Here's how the part is built. I have some questions about the finished solid (model axes, mm). Face numbers are marked on the shaded views. A direction names the side the tool comes from. Give positions to 0.01 mm unless a question says otherwise; leave off trailing zeros. Write each loop counter-clockwise with the first axis right and the second up, starting at its lowest first coordinate (ties: lowest second). Pieces come first, ordered by that corner, then holes. Notation, with made-up numbers: (64, 50.5) - (85, 50.5) arc R31 cw to (85, 78.5) - close; hole circle Ø4 at (51, 84). An arc over 180 degrees is marked (long way). Use a Markdown table: item, result.
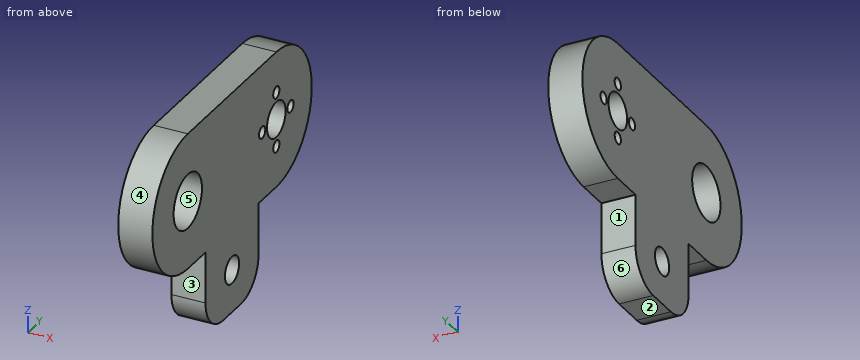
```python
from build123d import *

# Parameters (mm, degrees)
CROQUIS1_R              = 5.25
CROQUIS1_R_2            = 8
CROQUIS1_R_3            = 1.75
CROQUIS1_R_4            = 4
SALIENTE_EXTRUIR1_DEPTH = 10


with BuildPart() as part:
    # Croquis1 → Saliente-Extruir1 (new body)
    with BuildSketch(Plane(origin=(0, 0, 0), x_dir=(0, 0, -1), z_dir=(1, 0, 0))):
        with BuildLine():
            Line((20, 15), (20, 25))
            ThreePointArc((20, 25), (0, 45), (-20, 25))
            Line((-20, 25), (-20, -25))
            ThreePointArc((-20, -25), (0, -45), (20, -25))
            Line((20, -25), (20, -15))
            Line((20, -15), (35, -15))
            ThreePointArc((35, -15), (42.071067812, -12.071067812), (45, -5))
            Line((45, -5), (45, 5))
            ThreePointArc((45, 5), (42.071067812, 12.071067812), (35, 15))
            Line((35, 15), (20, 15))
        make_face()
        with Locations((0, 25)):
            Circle(CROQUIS1_R, mode=Mode.SUBTRACT)
        with Locations((0, -25)):
            Circle(CROQUIS1_R_2, mode=Mode.SUBTRACT)
        with Locations((0, 33)):
            Circle(CROQUIS1_R_3, mode=Mode.SUBTRACT)
        with Locations((8, 25)):
            Circle(CROQUIS1_R_3, mode=Mode.SUBTRACT)
        with Locations((0, 17)):
            Circle(CROQUIS1_R_3, mode=Mode.SUBTRACT)
        with Locations((-8, 25)):
            Circle(CROQUIS1_R_3, mode=Mode.SUBTRACT)
        with Locations((32.5, 0)):
            Circle(CROQUIS1_R_4, mode=Mode.SUBTRACT)
    extrude(amount=SALIENTE_EXTRUIR1_DEPTH)


solid = part.part
```
Item 1: If we section it at A-A, the plane y = 0: Write out the boundary of the cut face in (x, z).
Values:
| item | result |
|---|---|
| outline | (0, -45) - (10, -45) - (10, -36.5) - (0, -36.5) - close; (0, -28.5) - (10, -28.5) - (10, 20) - (0, 20) - close |
Item 2: I need wall thicknesses on line 1 along Y through (x, z) = (8, 0); line 2 along Z through (x, y) = (6.75, 16.5); line 3 along Z through (x, y) = (9, 29). Which ranges of each line are inside material? Lowest first, please. Write a range as [from, to].
Values:
| item | result |
|---|---|
| line 1 | y = [-45, -33], [-17, 15.25], [18.75, 19.75], [30.25, 31.25], [34.75, 45] |
| line 2 | z = [-20, -1.68], [1.68, 20] |
| line 3 | z = [-19.6, -3.4], [3.4, 19.6] |
Item 3: Will these pins go through, and if not, where does the flat tip stop? pin 1 Ø13 at (y, z) = (0, -32.5) entering from -X; pin 2 Ø2 at (x, y) = (8.5, -32) entering from +Z; pin 3 Ø4 at (x, z) = (2, 13) entering from -Y; pin 4 Ø5 at (x, y) = (3.5, 21) entering from -Z.
Values:
| item | result |
|---|---|
| pin 1 | stops at x = 0 |
| pin 2 | stops at z = 19.08 |
| pin 3 | stops at y = -41.7 |
| pin 4 | stops at z = -20 |
Item 4: If we section it at D-D, the plane z = -30.5: Write out the boundary of the cut face in (x, y).
Values:
| item | result |
|---|---|
| outline | (0, -15) - (10, -15) - (10, -3.46) - (0, -3.46) - close; (0, 3.46) - (10, 3.46) - (10, 15) - (0, 15) - close |
Item 5: For the marked faces 1, 2 and 3, which set-ups out of +Z, -Z, +X, -X, +Y, -Y let a thin tool reach every point of the face, with its end or its side?
Values:
| item | result |
|---|---|
| face 1 | -Z, +X, -X, +Y |
| face 2 | -Z, +X, -X, +Y, -Y |
| face 3 | -Z, +X, -X, -Y |
Item 6: If we section it at B-B, the plane z = 0: Write out the boundary of the cut face in (x, y), plus the area to 3 significant figures.
Values:
| item | result |
|---|---|
| outline | (0, -45) - (10, -45) - (10, -33) - (0, -33) - close; (0, -17) - (10, -17) - (10, 15.25) - (0, 15.25) - close; (0, 18.75) - (10, 18.75) - (10, 19.75) - (0, 19.75) - close; (0, 30.25) - (10, 30.25) - (10, 31.25) - (0, 31.25) - close; (0, 34.75) - (10, 34.75) - (10, 45) - (0, 45) - close |
| area | 565 mm2 |
Item 7: If we section it at C-C, the plane x = 6.75: Write out the boundary of the cut face in (y, z).
Values:
| item | result |
|---|---|
| outline | (-25, -20) - (-15, -20) - (-15, -35) arc R10 ccw to (-5, -45) - (5, -45) arc R10 ccw to (15, -35) - (15, -20) - (25, -20) arc R20 ccw to (25, 20) - (-25, 20) arc R20 ccw to start; hole circle Ø16 at (-25, 0); hole circle Ø8 at (0, -32.5); hole circle Ø3.5 at (17, 0); hole circle Ø10.5 at (25, 0); hole circle Ø3.5 at (25, -8); hole circle Ø3.5 at (25, 8); hole circle Ø3.5 at (33, 0) |
Item 8: Thinking about a two-plate mould opening in Y: for the marked faces 4, 5 and 6, which applies, +Y half, -Y half, draft (parallel to the pull), parting line (faces both ways), or undercut?
Values:
| item | result |
|---|---|
| face 4 | -Y half |
| face 5 | undercut |
| face 6 | +Y half |
